Input: part model. Units: mm. Frame: model coordinates. Face numbers are marked on the shaded views. A direction names the side the tool comes from. Coordinates: 2 decimals unless noted, no trailing zeros. Write each loop counter-clockwise with the first axis right and the second up, starting at its lowest first coordinate (ties: lowest second). Pieces come first, ordered by that corner, then holes.
from build123d import *

# Parameters (mm, degrees)
SKETCH1_R           = 6.05
BOSS_EXTRUDE1_DEPTH = 10
SKETCH1_3_R         = 7.55
BOSS_EXTRUDE2_DEPTH = 4
BOSS_EXTRUDE3_START = 4
SKETCH1_5_R         = 8.55
SKETCH1_5_R_2       = 7.55
SKETCH1_5_R_3       = 6.05
BOSS_EXTRUDE3_DEPTH = 2.5


with BuildPart() as part:
    # Sketch1 → Boss-Extrude1 (new body)
    with BuildSketch(Plane(origin=(0, 0, 0), x_dir=(1, 0, 0), z_dir=(0, 1, 0))):
        with Locations(Location((0, 0, 0), (0, 0, 270))):
            Circle(SKETCH1_R)
        Polygon((5.773502692, 0), (2.886751346, 5), (-2.886751346, 5), (-5.773502692, 0), (-2.886751346, -5), (2.886751346, -5), align=None, mode=Mode.SUBTRACT)
    extrude(amount=-BOSS_EXTRUDE1_DEPTH)

    # Sketch1<3> → Boss-Extrude2 (add)
    with BuildSketch(Plane(origin=(0, 0, 0), x_dir=(1, 0, 0), z_dir=(0, 1, 0))):
        with Locations(Location((1.5, 0, 0), (0, 0, 180))):
            Circle(SKETCH1_3_R)
        Polygon((2.886751346, 5), (-2.886751346, 5), (-5.773502692, 0), (-2.886751346, -5), (2.886751346, -5), (5.773502692, 0), align=None, mode=Mode.SUBTRACT)
    extrude(amount=BOSS_EXTRUDE2_DEPTH)

    # Sketch1<5> → Boss-Extrude3 (add)
    # profile 1 of 3: a face of its own
    with BuildSketch(Plane(origin=(0, 0, 0), x_dir=(1, 0, 0), z_dir=(0, 1, 0)).offset(BOSS_EXTRUDE3_START)):
        with Locations(Location((1.5, 0, 0), (0, 0, 270))):
            Circle(SKETCH1_5_R)
        with Locations(Location((1.5, 0, 0), (0, 0, 180))):
            Circle(SKETCH1_5_R_2, mode=Mode.SUBTRACT)
    # profile 2 of 3: a face of its own
    with BuildSketch(Plane(origin=(0, 0, 0), x_dir=(1, 0, 0), z_dir=(0, 1, 0)).offset(BOSS_EXTRUDE3_START)):
        with Locations(Location((1.5, 0, 0), (0, 0, 180))):
            Circle(SKETCH1_5_R_2)
        with Locations(Location((0, 0, 0), (0, 0, 270))):
            Circle(SKETCH1_5_R_3, mode=Mode.SUBTRACT)
    # profile 3 of 3: a face of its own
    with BuildSketch(Plane(origin=(0, 0, 0), x_dir=(1, 0, 0), z_dir=(0, 1, 0)).offset(BOSS_EXTRUDE3_START)):
        with Locations(Location((0, 0, 0), (0, 0, 270))):
            Circle(SKETCH1_5_R_3)
        Polygon((5.773502692, 0), (2.886751346, 5), (-2.886751346, 5), (-5.773502692, 0), (-2.886751346, -5), (2.886751346, -5), align=None, mode=Mode.SUBTRACT)
    extrude(amount=BOSS_EXTRUDE3_DEPTH)


solid = part.part
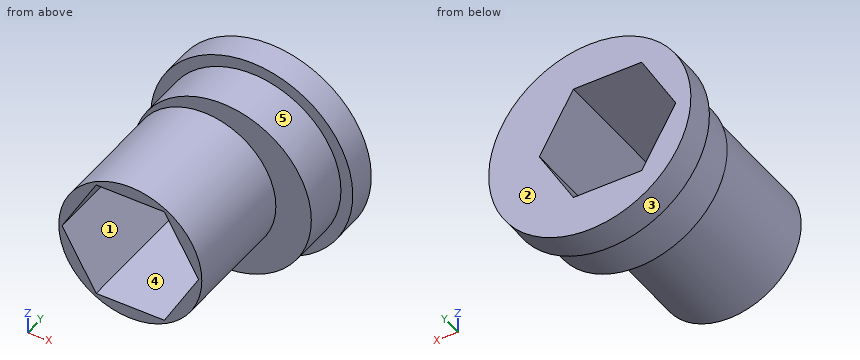
Item 1: Pull-direction query (Z, two-part tool) for the marked faces 1, 2 and 3; classes: released by +Z, released by -Z, zero draft, split by the parting line, or undercut.
Item 2: Material intervals for line 1 (Y direction, x = -4, z = 6.5); line 2 (Z direction, x = -2.75, y = 5); line 3 (Y direction, x = 8, z = 0.5), sorted ascending.
Item 3: Section query B-B, the plane y = 5.5. Return loops of the section in (x, z), then the cut area to 3 significant figures.
Item 4: Pin query (flat end, axial travel): pin 1 Ø1 at (x, y) = (2.5, 4) entering from +Z; pin 2 Ø5 at (x, y) = (-3.5, 0.5) entering from -Z; pin 3 Ø3 at (x, y) = (1, -5.5) entering from -Z. Return the tip coordinate at first contact, or that it passes through.
Item 5: Section query D-D, the plane y = -2. Return loops of the section in (x, z), then the cut area to 3 significant figures.
Item 6: Section query C-C, the plane z = -3.25. Return loops of the section in (x, y).
Item 7: Section query A-A, the plane x = 3.75. Return loops of the section in (y, z).
Item 8: Access query for the marked faces 4 and 5. Directions: +Z, -Z, +X, -X, +Y, -Y. A direction counts if a zero-diameter tool reaches every point of the face in a straight line with its end or side. Return the directions, or none.
The answers:
1. face 1: undercut
1. face 2: zero draft
1. face 3: split by the parting line
2. line 1: y = 4 to 6.5
2. line 2: z = -7.42 to -5, 5 to 7.42
2. line 3: y = 0 to 6.5
3. outline: circle Ø17.1 at (1.5, 0); hole (-5.77, 0) - (-2.89, -5) - (2.89, -5) - (5.77, 0) - (2.89, 5) - (-2.89, 5) - close
3. area: 143 mm2
4. pin 1: stops at z = 8.54
4. pin 2: stops at z = -7.12
4. pin 3: stops at z = -6.05
5. outline: circle Ø12.1 at (0, 0); hole (-5.77, 0) - (-2.89, -5) - (2.89, -5) - (5.77, 0) - (2.89, 5) - (-2.89, 5) - close
5. area: 28.4 mm2
6. outline: (-6.41, 4) - (-5.31, 4) - (-5.31, 0) - (-5.1, 0) - (-5.1, -10) - (-3.9, -10) - (-3.9, 6.5) - (-6.41, 6.5) - close; (3.9, -10) - (5.1, -10) - (5.1, 0) - (8.31, 0) - (8.31, 4) - (9.41, 4) - (9.41, 6.5) - (3.9, 6.5) - close
7. outline: (-10, -4.75) - (0, -4.75) - (0, -7.21) - (4, -7.21) - (4, -8.25) - (6.5, -8.25) - (6.5, -3.5) - (-10, -3.5) - close; (-10, 3.5) - (6.5, 3.5) - (6.5, 8.25) - (4, 8.25) - (4, 7.21) - (0, 7.21) - (0, 4.75) - (-10, 4.75) - close
8. face 4: +Y, -Y
8. face 5: -Y
